```python
from build123d import *

# Parameters (mm, degrees)
SKETCH1_W           = 151.015799324
SKETCH1_H           = 90.161719468
BOSS_EXTRUDE1_DEPTH = 10
SKETCH2_R           = 4.522511264
CUT_EXTRUDE1_DEPTH  = 10
TPATTERN1_START     = 5
TPATTERN1_OUTLINE_R = 4.522511264
TPATTERN1_DEPTH     = 5


# Read off the part's stored shape, not the designer's step: TPattern1
with BuildPart() as part:
    # Sketch1 → Boss-Extrude1 (new body)
    with BuildSketch(Plane(origin=(0, 0, 0), x_dir=(1, 0, 0), z_dir=(0, 1, 0))):
        with Locations((4.769946885, -6.090262952)):
            Rectangle(SKETCH1_W, SKETCH1_H)
    extrude(amount=BOSS_EXTRUDE1_DEPTH)

    # Sketch2 → Cut-Extrude1 (cut)
    with BuildSketch(Plane(origin=(0, 10, 0), x_dir=(-1, 0, 0), z_dir=(0, 1, 0))):
        with Locations(Location((56.686327356, 33.019898718, 0), (0, 0, 90))):
            Circle(SKETCH2_R)
    extrude(amount=-CUT_EXTRUDE1_DEPTH, mode=Mode.SUBTRACT)

    # TPattern1 outline → TPattern1 (cut)
    with BuildSketch(Plane(origin=(0, 0, 0), x_dir=(1, 0, 0), z_dir=(0, 1, 0)).offset(TPATTERN1_START)):
        with Locations((-56.686327356, -16.090262952)):
            Circle(TPATTERN1_OUTLINE_R)
        with Locations((-56.686327356, 23.909737048)):
            Circle(TPATTERN1_OUTLINE_R)
    extrude(amount=TPATTERN1_DEPTH, mode=Mode.SUBTRACT)


solid = part.part
```
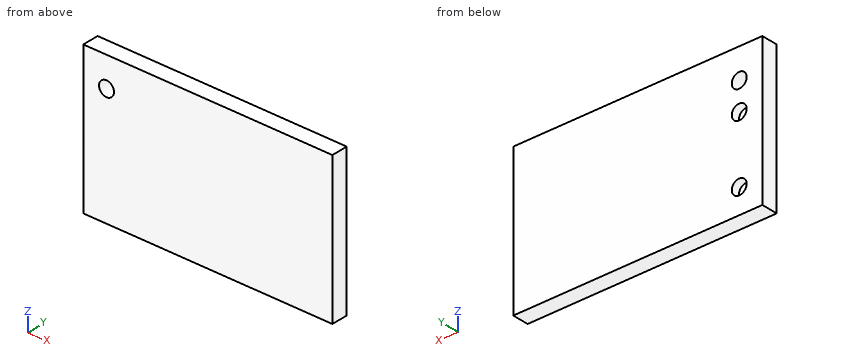
The listing builds one solid part. Answer for the finished solid, in the listing's coordinates (mm). Round coordinates to 2 decimals unless told otherwise and drop trailing zeros. Loops run counter-clockwise (first coordinate to the right, second up) from the corner with the lowest first, then second, coordinate; pieces in that order, holes last.
Q1. Given pin 1 Ø2.5 at (x, z) = (-59, -25.5) entering from +Y, flat-ended and moving along its own axis, determine where the tip first touches the part or whether it passes through.
Q2. Section B-B, the plane z = 19 is taken. Determine the outline of the cut face in (x, y).
Q3. Find the intervals of material crossed by line 1 (X direction, y = 5.5, z = -24); line 2 (X direction, y = 8, z = -28); line 3 (Z direction, x = -56, y = 1.25), in increasing order.
Q4. Section C-C, the plane z = -22 is taken. Determine the outline of the cut face in (x, y), then the cut area to 3 significant figures.
Q5. Section A-A, the plane z = 32 is taken. Determine the outline of the cut face in (x, y).
Completed:
1. pin 1: stops at y = 5
2. outline: (-70.74, 0) - (80.28, 0) - (80.28, 10) - (-53.22, 10) - (-53.22, 5) - (-60.15, 5) - (-60.15, 10) - (-70.74, 10) - close
3. line 1: x = -70.74 to -61.21, -52.16 to 80.28
3. line 2: x = -70.74 to -58.62, -54.76 to 80.28
3. line 3: z = -38.99 to 28.55, 37.49 to 51.17
4. outline: (-70.74, 0) - (80.28, 0) - (80.28, 10) - (-52.59, 10) - (-52.59, 5) - (-60.79, 5) - (-60.79, 10) - (-70.74, 10) - close
4. area: 1,470 mm2
5. outline: (-70.74, 0) - (-61.09, 0) - (-61.09, 10) - (-70.74, 10) - close; (-52.28, 0) - (80.28, 0) - (80.28, 10) - (-52.28, 10) - close
